Drawing for the job (mm, zero at the part's lowest x, y, z). Coordinates: 2 decimals unless noted, no trailing zeros. Order: outer loops, then holes, each group sorted by start corner. A loop starts at its lowest first (then second) coordinate and runs counter-clockwise, first axis right, second up. Notation, with made-up numbers: (2, 25) - (42, 25) arc R11 cw to (42, 41) - close; hole circle Ø1 at (5.5, 43). An arc over 180 degrees is marked (long way). Answer as CSV lines item,"result". Start each with the question number.
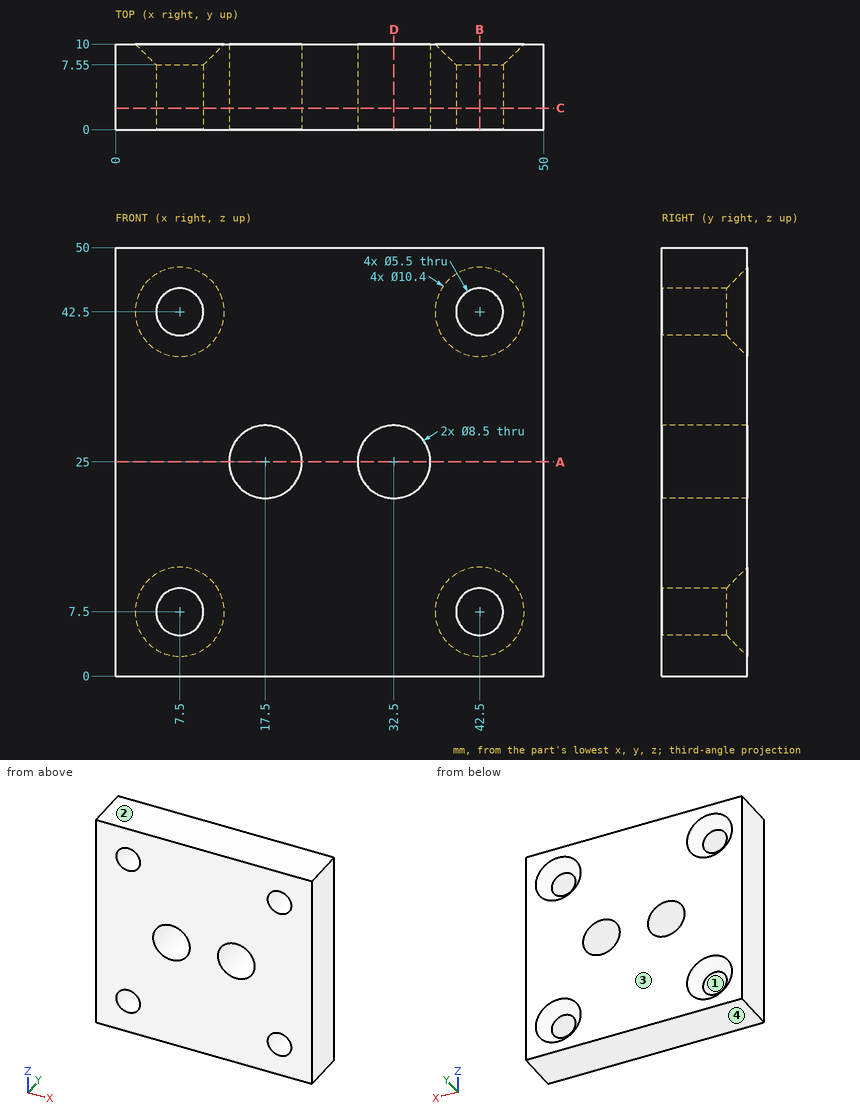
(1) Drop flat-ended pins along their axis: pin 1 Ø2 at (x, y) = (10, 3.5) entering from -Z; pin 2 Ø7 at (x, z) = (42.5, 7.5) entering from +Y. Give the stop position or say it passes through.
(2) Band-saw the part on B-B on x = 42.5. List the corners of the cut face in (y, z), plus the area to 3 significant figures.
(3) Pull direction Z, two halves, no side cores. Call the marked faces 1, 2, 3 and 4: +Z half, -Z half, draft (parallel to the pull), parting line (faces both ways), or undercut.
(4) Probe L1, parallel to Z at x = 42.5, y = 5.5; L2, parallel to Z at x = 32.5, y = 6. List the from-to ranges inside material, lowest first. Write a range as [from, to].
(5) Band-saw the part on D-D on x = 32.5. List the corners of the cut face in (y, z), plus the area to 3 significant figures.
(6) Band-saw the part on C-C on y = 2.5. List the corners of the cut face in (x, z).
(7) Band-saw the part on A-A on z = 25. List the corners of the cut face in (x, y).
Filled in:
1,pin 1,"stops at z = 0"
1,pin 2,"stops at y = 8.3"
2,outline,"(0, 0) - (10, 0) - (10, 2.3) - (7.55, 4.75) - (0, 4.75) - close; (0, 10.25) - (7.55, 10.25) - (10, 12.7) - (10, 37.3) - (7.55, 39.75) - (0, 39.75) - close; (0, 45.25) - (7.55, 45.25) - (10, 47.7) - (10, 50) - (0, 50) - close"
2,area,"378 mm^2"
3,face 1,"undercut"
3,face 2,"+Z half"
3,face 3,"draft"
3,face 4,"-Z half"
4,L1,"z = [0, 4.75], [10.25, 39.75], [45.25, 50]"
4,L2,"z = [0, 20.75], [29.25, 50]"
5,outline,"(0, 0) - (10, 0) - (10, 20.75) - (0, 20.75) - close; (0, 29.25) - (10, 29.25) - (10, 50) - (0, 50) - close"
5,area,"415 mm^2"
6,outline,"(0, 0) - (50, 0) - (50, 50) - (0, 50) - close; hole circle Ø5.5 at (7.5, 7.5); hole circle Ø5.5 at (7.5, 42.5); hole circle Ø8.5 at (17.5, 25); hole circle Ø8.5 at (32.5, 25); hole circle Ø5.5 at (42.5, 7.5); hole circle Ø5.5 at (42.5, 42.5)"
7,outline,"(0, 0) - (13.25, 0) - (13.25, 10) - (0, 10) - close; (21.75, 0) - (28.25, 0) - (28.25, 10) - (21.75, 10) - close; (36.75, 0) - (50, 0) - (50, 10) - (36.75, 10) - close"
